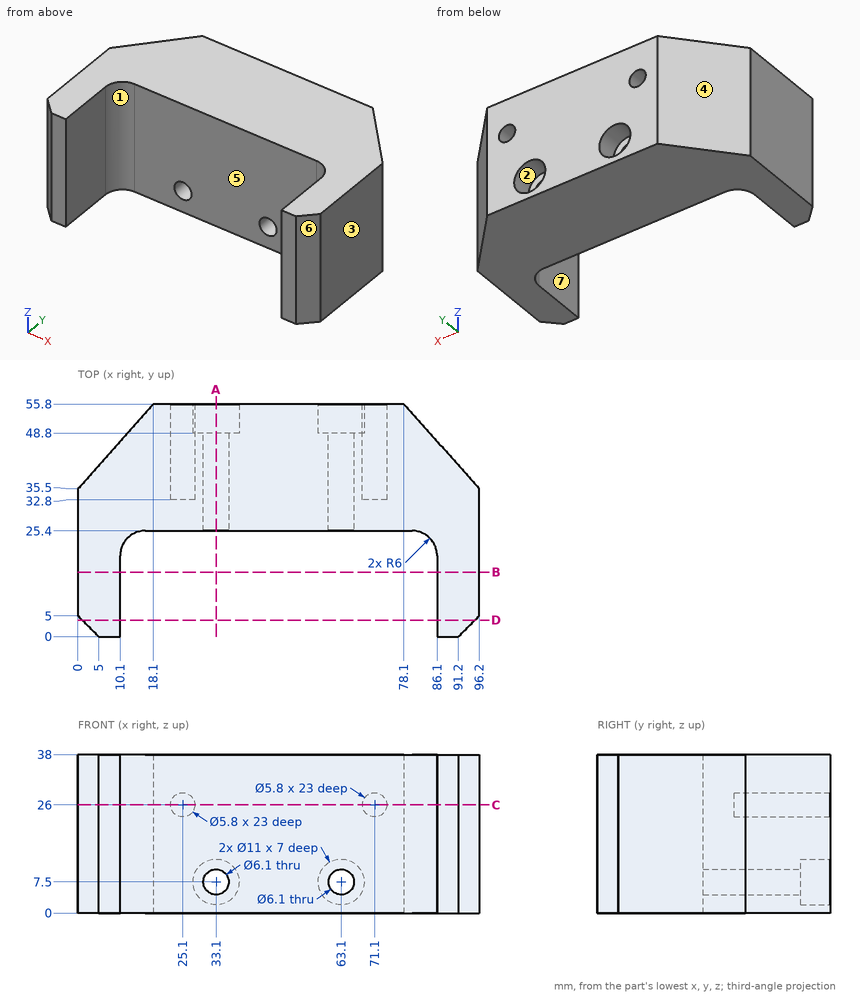
Can you work these out from the drawing? Everything is in mm from the part's minimum corner. A direction names the side the tool comes from. Give positions to 0.01 mm unless a question says otherwise; leave off trailing zeros. Loops run counter-clockwise (first coordinate to the right, second up) from the corner with the lowest first, then second, coordinate; pieces in that order, holes last. Notation, with made-up numbers: M 59,9.25 L 79,9.25 A31 ccw 79,40.25 Z; hole C 33.25,36 d7. An arc over 180 degrees is marked long. Use CSV: the item, a comma, the result in double quotes. Start each with the question number.
1. On a 3-axis mill with a long thin cutter (end or side, diameter ignored), from which of +Z, -Z, +X, -X, +Y, -Y can I reach the whole of each face in a straight line? I mean the marked faces 1, 2 and 3. Say none if no direction works.
2. Imagine slicing it at A-A, the plane x = 33.1. Write out the boundary of the cut face in (y, z).
3. Imagine slicing it at D-D, the plane y = 4. Write out the boundary of the cut face in (x, z).
4. For P1, Ø5, axis at y = 45, z = 4, coming from the -X side; P2, Ø8, axis at x = 22.5, z = 5, coming from the -Y side; P3, Ø1, axis at x = 84, y = 14.5, coming from the -Z side; P4, Ø10, axis at x = 63.1, z = 7.5, coming from the +Y side, each with a flat end and sliding along its axis, tell me the tip position at first contact or that it passes through.
5. Imagine slicing it at B-B, the plane y = 15.5. Write out the boundary of the cut face in (x, z).
6. If we mould it in two halves opening along X, with no side actions, what happens to the marked faces 4, 5, 6 and 7? For each: released by +X, released by -X, zero draft, split by the parting line, or undercut.
7. Imagine slicing it at C-C, the plane z = 26. Write out the boundary of the cut face in (x, y).
8. If I drill on L1, parallel to Z at x = 33, y = 50; L2, parallel to Z at x = 25.1, y = 41.25; L3, parallel to X at y = 11, z = 36, over which ranges is the centre line in solid material (lowest first)?
Response values:
1,face 1,"+Z, -Z, -Y"
1,face 2,"+Y"
1,face 3,"+Z, -Z, +X, +Y, -Y"
2,outline,"M 25.4,0 L 55.8,0 L 55.8,2 L 48.8,2 L 48.8,4.45 L 25.4,4.45 Z; M 25.4,10.55 L 48.8,10.55 L 48.8,13 L 55.8,13 L 55.8,38 L 25.4,38 Z"
3,outline,"M 1,0 L 10.1,0 L 10.1,38 L 1,38 Z; M 86.1,0 L 95.2,0 L 95.2,38 L 86.1,38 Z"
4,P1,"x = 6.24"
4,P2,"y = 25.4"
4,P3,"through"
4,P4,"y = 48.8"
5,outline,"M 0,0 L 10.1,0 L 10.1,38 L 0,38 Z; M 86.1,0 L 96.2,0 L 96.2,38 L 86.1,38 Z"
6,face 4,"released by -X"
6,face 5,"undercut"
6,face 6,"released by +X"
6,face 7,"undercut"
7,outline,"M 0,5 L 5,0 L 10.1,0 L 10.1,19.4 A6 cw 16.1,25.4 L 80.1,25.4 A6 cw 86.1,19.4 L 86.1,0 L 91.2,0 L 96.2,5 L 96.2,35.5 L 78.1,55.8 L 74,55.8 L 74,32.8 L 68.2,32.8 L 68.2,55.8 L 28,55.8 L 28,32.8 L 22.2,32.8 L 22.2,55.8 L 18.1,55.8 L 0,35.5 Z"
8,L1,"0 to 2, 13 to 38"
8,L2,"0 to 23.1, 28.9 to 38"
8,L3,"0 to 10.1, 86.1 to 96.2"
